Could you check a few things on this model? Use its own coordinates, in mm. A direction names the side the tool comes from. Round coordinates to 2 decimals unless told otherwise and drop trailing zeros. Write each loop counter-clockwise with the first axis right and the second up, starting at its lowest first coordinate (ties: lowest second). Pieces come first, ordered by that corner, then holes. Notation, with made-up numbers: M 14.5,-18.75 L 20.5,-18.75 A5 ccw 20.5,-9.75 Z; hole C -7.75,52 d1. An arc over 180 degrees is marked long. One line per item, written item: value. Start each with the question number.
(1) I want a section at B-B on x = -8. Please give me the cut outline in (y, z).
(2) If I drill on L1, parallel to X at y = -18.5, z = -12.5; L2, parallel to Y at x = 33.5, z = -4.75; L3, parallel to Y at x = -50.5, z = -9.75, over which ranges is the centre line in solid material (lowest first)?
(3) I want a section at D-D on y = 22. Please give me the cut outline in (x, z), and give its area (3 significant figures).
(4) I want a section at C-C on z = -11.75. Count the separate pieces of the cut face and the enclosed holes in it, and give its area (3 significant figures).
(5) Thinking about a two-plate mould opening in Y: for faces 1 (the face through (-4, 33.942, -24)), 2 (the face through (-4, 34.892, -13)), 3 (the face through (50.646, -1, -13)), which applies, released by +Y, released by -Y, zero draft, split by the parting line, or undercut?
(6) Which directions (+Z, -Z, +X, -X, +Y, -Y) give clear straight access to the entire face, cutting with the end or side of a thin tool? Please do faces 4 (the face through (41, -34.158, -24)), 5 (the face through (50, 0, -25)), 6 (the face through (-3, -14.108, -1)).
(7) I want a section at A-A on y = 2. Please give me the cut outline in (x, z).
(8) I'm going to push flat-ended pins straight in: pin 1 Ø6.5 at (x, y) = (-50.5, -27.5) entering from -Z; pin 2 Ø12 at (x, y) = (-3, 14.5) entering from -Z; pin 3 Ø0.5 at (y, z) = (34.5, -24) entering from +X; pin 4 Ø1.6 at (x, z) = (-20, -1) entering from -Y. Where does each tip first touch, or does it pass through?
```python
from build123d import *

# Parameters (mm, degrees)
F0_W      = 108
F0_H      = 70
F0_W_2    = 106.1
F0_H_2    = 68.1
F0_W_3    = 104
F0_H_3    = 66
F0_R      = 3
F1_DEPTH  = 2
F2_DEPTH  = 22.49
F3_DEPTH  = 23
F4_DEPTH  = 14
F6_DEPTH  = 2.5
F7_W      = 21
F7_H      = 2.4
F8_DEPTH  = 2.5
F10_D     = 2.4384
F10_DEPTH = 10
F10_TIP   = 0.7325692667
F11_R     = 1.5
F12_R     = 1.5


with BuildPart() as f1:
    # F0 (on Top) → F1 (new body)
    with BuildSketch(Plane.XY):
        with Locations((-3.3541592062, -0.1079301417)):
            Rectangle(F0_W, F0_H)
        with Locations((-3.3541592062, -0.1079301417)):
            Rectangle(F0_W_2, F0_H_2, mode=Mode.SUBTRACT)
        with Locations((-3.3541592062, -0.1079301417)):
            Rectangle(F0_W_2, F0_H_2)
        with Locations((-3.3541592062, -0.1079301417)):
            Rectangle(F0_W_3, F0_H_3, mode=Mode.SUBTRACT)
        with Locations((-3.3541592062, -0.1079301417)):
            Rectangle(F0_W_3, F0_H_3)
        with Locations((-49.8541592062, -27.6079301417)):
            Circle(F0_R, mode=Mode.SUBTRACT)
        with Locations((43.1458407938, -27.6079301417)):
            Circle(F0_R, mode=Mode.SUBTRACT)
        with Locations((-49.8541592062, 27.3920698583)):
            Circle(F0_R, mode=Mode.SUBTRACT)
        with BuildLine():
            ThreePointArc((-43.3541592062, 13.4650188752), (-44.1826393193, 16.2812101433), (-41.2730203761, 15.8920698583))
            Line((-41.2730203761, 15.8920698583), (34.5647019638, 15.8920698583))
            ThreePointArc((34.5647019638, 15.8920698583), (36.5302279992, 16.8493327192), (37.8958407938, 15.1420698583))
            ThreePointArc((37.8958407938, 15.1420698583), (37.5489623139, 14.0962448251), (36.6458407938, 13.4650188752))
            Line((36.6458407938, 13.4650188752), (36.6458407938, -11.6808791586))
            ThreePointArc((36.6458407938, -11.6808791586), (37.5489623139, -12.3121051085), (37.8958407938, -13.3579301417))
            ThreePointArc((37.8958407938, -13.3579301417), (36.5302279992, -15.0651930026), (34.5647019638, -14.1079301417))
            Line((34.5647019638, -14.1079301417), (-41.2730203761, -14.1079301417))
            ThreePointArc((-41.2730203761, -14.1079301417), (-44.1826393193, -14.4970704267), (-43.3541592062, -11.6808791586))
            Line((-43.3541592062, -11.6808791586), (-43.3541592062, 13.4650188752))
        make_face(mode=Mode.SUBTRACT)
        with Locations((43.1458407938, 27.3920698583)):
            Circle(F0_R, mode=Mode.SUBTRACT)
        with Locations((-49.8541592062, 27.3920698583)):
            Circle(F0_R)
        with Locations((43.1458407938, 27.3920698583)):
            Circle(F0_R)
        with Locations((43.1458407938, -27.6079301417)):
            Circle(F0_R)
        with Locations((-49.8541592062, -27.6079301417)):
            Circle(F0_R)
    extrude(amount=-F1_DEPTH)

    # F0 (on Top) → F2 (join)
    with BuildSketch(Plane.XY):
        with Locations((-3.3541592062, -0.1079301417)):
            Rectangle(F0_W_2, F0_H_2)
        with Locations((-3.3541592062, -0.1079301417)):
            Rectangle(F0_W_3, F0_H_3, mode=Mode.SUBTRACT)
    extrude(amount=-F2_DEPTH)

    # F3 (add): a face of the model
    f3_faces = [f1.faces().sort_by_distance(p)[0] for p in [
        (50.5171395895, -0.1079301417, -2),
    ]]
    extrude(f3_faces, amount=F3_DEPTH)

    # F0 (on Top) → F4 (join)
    with BuildSketch(Plane.XY):
        with Locations((-49.8541592062, 27.3920698583)):
            Circle(F0_R)
        with Locations((43.1458407938, 27.3920698583)):
            Circle(F0_R)
        with Locations((-49.8541592062, -27.6079301417)):
            Circle(F0_R)
        with Locations((43.1458407938, -27.6079301417)):
            Circle(F0_R)
    extrude(amount=-F4_DEPTH)

    # F5 (on face) → F6 (cut)
    with BuildSketch(Plane.XZ.offset(35.1079301417)):
        with BuildLine():
            Line((19.1458407938, -25), (32.1458407938, -25))
            ThreePointArc((32.1458407938, -25), (25.6458407938, -18.5), (19.1458407938, -25))
        make_face()
    extrude(amount=-F6_DEPTH, mode=Mode.SUBTRACT)

    # F7 (on face) → F8 (cut)
    with BuildSketch(Plane(origin=(0, 34.8920698583, 0), x_dir=(-1, 0, 0), z_dir=(0, 1, 0))):
        with Locations((-18.5458407938, -23.8)):
            Rectangle(F7_W, F7_H)
    extrude(amount=-F8_DEPTH, mode=Mode.SUBTRACT)

    # F10
    with Locations(Plane(origin=(0, 0, -14), x_dir=(1, 0, 0), z_dir=(0, 0, -1))):
        with Locations((-49.8525463045, -27.2346809506), (43.3072187006, -27.4257659912), (43.1458407938, 27.6079301417), (-49.7261881828, 27.6079301417)):
            Hole(F10_D / 2, depth=F10_DEPTH)
            with Locations((0, 0, -(F10_DEPTH + F10_TIP / 2))):  # 118° drill point
                Cone(0, F10_D / 2, F10_TIP, mode=Mode.SUBTRACT)

    # F11
    f11_edges = [f1.edges().sort_by_distance(p)[0] for p in [
        (-57.354159, -0.10793, 0),
        (-3.354159, 34.89207, 0),
        (50.645841, -0.10793, 0),
        (50.645841, -35.10793, -12.5),
        (-3.354159, -35.10793, 0),
        (-57.354159, -35.10793, -12.5),
        (50.645841, 34.89207, -12.5),
        (-57.354159, 34.89207, -12.5),
    ]]
    fillet(f11_edges, radius=F11_R)

    # F12
    f12_edges = [f1.edges().sort_by_distance(p)[0] for p in [
        (48.645841, -33.10793, -12.245),
        (48.645841, -0.10793, -2),
        (-3.354159, -33.10793, -2),
        (-55.354159, -33.10793, -12.245),
        (-55.354159, -0.10793, -2),
        (-55.354159, 32.89207, -12.245),
        (-3.354159, 32.89207, -2),
        (48.645841, 32.89207, -12.245),
    ]]
    fillet(f12_edges, radius=F12_R)


solid = f1.part
```
Found:
1. outline: M -35.11,-25 L -34.16,-25 L -34.16,-22.49 L -33.11,-22.49 L -33.11,-3.5 A1.5 cw -31.61,-2 L -14.11,-2 L -14.11,0 L -33.61,0 A1.5 ccw -35.11,-1.5 Z; M 15.89,-2 L 31.39,-2 A1.5 cw 32.89,-3.5 L 32.89,-22.49 L 33.94,-22.49 L 33.94,-25 L 34.89,-25 L 34.89,-1.5 A1.5 ccw 33.39,0 L 15.89,0 Z
2. L1: x = -57.35 to -55.35, 48.65 to 50.65
2. L2: y = -35.11 to -33.11, 32.89 to 34.89
2. L3: y = -35.11 to -33.11, -30.54 to -28.55, -26.67 to -24.68, 24.46 to 26.2, 28.27 to 30.32, 32.89 to 34.89
3. outline: M -57.35,-25 L -56.4,-25 L -56.4,-22.49 L -55.35,-22.49 L -55.35,-3.5 A1.5 cw -53.85,-2 L 47.15,-2 A1.5 cw 48.65,-3.5 L 48.65,-22.49 L 49.7,-22.49 L 49.7,-25 L 50.65,-25 L 50.65,-1.5 A1.5 ccw 49.15,0 L -55.85,0 A1.5 ccw -57.35,-1.5 Z
3. area: 303 mm²
4. separate pieces: 5
4. enclosed holes: 5
4. area: 790 mm²
5. face 1: undercut
5. face 2: released by +Y
5. face 3: zero draft
6. face 4: -Z
6. face 5: -Z, +X, -X, +Y, -Y
6. face 6: +Z, -Z
7. outline: M -57.35,-25 L -56.4,-25 L -56.4,-22.49 L -55.35,-22.49 L -55.35,-3.5 A1.5 cw -53.85,-2 L -43.35,-2 L -43.35,0 L -55.85,0 A1.5 ccw -57.35,-1.5 Z; M 36.65,-2 L 47.15,-2 A1.5 cw 48.65,-3.5 L 48.65,-22.49 L 49.7,-22.49 L 49.7,-25 L 50.65,-25 L 50.65,-1.5 A1.5 ccw 49.15,0 L 36.65,0 Z
8. pin 1: stops at z = -14
8. pin 2: stops at z = -2
8. pin 3: stops at x = 50.38
8. pin 4: stops at y = -35.11
